Verification items for the finished model (mm, model axes). A direction names the side the tool comes from. Give positions to 0.01 mm unless a question says otherwise; leave off trailing zeros. Write each loop counter-clockwise with the first axis right and the second up, starting at its lowest first coordinate (ties: lowest second). Pieces come first, ordered by that corner, then holes. Notation, with made-up numbers: (57, -37) - (98, -37) arc R22 ccw to (98, -8) - close; hole circle Ø6 at (31, 42.25). An arc over 180 degrees is marked (long way). Put each result on its own line as item: value.
from build123d import *

# Parameters (mm, degrees)
BASPROSKE_W         = 6
BASPROSKE_H         = 8
TOOTHCUT_DEPTH      = 13.806248475
TEETHCUTS_COUNT     = 14
TEETHCUTS_ANGLE     = 334.285714286
BORSKE_R            = 2.5
BORE_DEPTH          = 50.0000508
SKETCH1_R           = 2.5
BOSS_EXTRUDE1_DEPTH = 2.5
SKETCH2_R           = 2.5
CUT_EXTRUDE1_DEPTH  = 1.5
SKETCH3_R           = 1.1
CUT_EXTRUDE2_DEPTH  = 13.073146116


with BuildPart() as part:
    # BasProSke → Base-Revolve (revolve)
    with BuildSketch(Plane(origin=(0, 0, 0), x_dir=(1, 0, 0), z_dir=(0, 1, 0)), mode=Mode.PRIVATE) as base_revolve_sk:
        with Locations((3, 4)):
            Rectangle(BASPROSKE_W, BASPROSKE_H)
    revolve(base_revolve_sk.sketch.rotate(Axis((-10, 0, 0), (1, 0, 0)), 180), axis=Axis((-10, 0, 0), (1, 0, 0)))

    # TooCutSke → ToothCut (cut, through all)
    with BuildSketch(Plane(origin=(0, 0, 0), x_dir=(0, 0, -1), z_dir=(1, 0, 0))):
        with BuildLine():
            ThreePointArc((0.540393256, 5.723545765), (0, 5.749), (-0.540393256, 5.723545765))
            ThreePointArc((-0.540393256, 5.723545765), (-0.832220085, 6.912663993), (-1.603550271, 7.863566092))
            ThreePointArc((-1.603550271, 7.863566092), (0, 8.0254), (1.603550271, 7.863566092))
            ThreePointArc((1.603550271, 7.863566092), (0.832220085, 6.912663993), (0.540393256, 5.723545765))
        make_face()
    toothcut = extrude(amount=TOOTHCUT_DEPTH, mode=Mode.SUBTRACT)

    # TeethCuts: ToothCut ×14 about axis
    teethcuts_axis = Axis((-10, 0, 0), (1, 0, 0))
    for i in range(1, TEETHCUTS_COUNT):
        add(toothcut.rotate(teethcuts_axis, i * TEETHCUTS_ANGLE / (TEETHCUTS_COUNT - 1)), mode=Mode.SUBTRACT)

    # BorSke → Bore (cut, symmetric)
    with BuildSketch(Plane(origin=(0, 0, 0), x_dir=(0, 0, -1), z_dir=(1, 0, 0))):
        with Locations(Location((0, 0, 0), (0, 0, 180))):
            Circle(BORSKE_R)
    extrude(amount=BORE_DEPTH, both=True, mode=Mode.SUBTRACT)

    # Sketch1 → Boss-Extrude1 (add)
    with BuildSketch(Plane(origin=(6, 0, 0), x_dir=(0, 0, -1), z_dir=(1, 0, 0))):
        Circle(SKETCH1_R)
    extrude(amount=-BOSS_EXTRUDE1_DEPTH)

    # Sketch2 → Cut-Extrude1 (cut)
    with BuildSketch(Plane(origin=(6, 0, 0), x_dir=(0, 0, -1), z_dir=(1, 0, 0))):
        Circle(SKETCH2_R)
    extrude(amount=-CUT_EXTRUDE1_DEPTH, mode=Mode.SUBTRACT)

    # Sketch3 → Cut-Extrude2 (cut, through all)
    with BuildSketch(Plane(origin=(4.5, 0, 0), x_dir=(0, 0, -1), z_dir=(1, 0, 0))):
        Circle(SKETCH3_R)
    extrude(amount=-CUT_EXTRUDE2_DEPTH, mode=Mode.SUBTRACT)


solid = part.part
Q1. Scan lines: line 1 along Y through (x, z) = (1.8, 7.25); line 2 along Z through (x, y) = (1.5, 0); line 3 along Z through (x, y) = (1.75, 5.25). Record each from-to range of solid material in increasing order.
Answers follow:
line 1: y = -3.38 to -3.2, -0.63 to 0.63, 3.2 to 3.38
line 2: z = -8 to -2.5, 2.5 to 8
line 3: z = -5 to -3.17, -2.34 to 2.34, 3.17 to 5
Q2. Section check D-D, the plane y = -2. Record the cut outline in (x, z), plus the area to 3 significant figures.
Answers follow:
outline: (0, -6.01) - (6, -6.01) - (6, -1.5) - (4.5, -1.5) - (4.5, 1.5) - (6, 1.5) - (6, 6.01) - (0, 6.01) - (0, 1.5) - (3.5, 1.5) - (3.5, -1.5) - (0, -1.5) - close
area: 57.1 mm2
Q3. Section check B-B, the plane z = 0. Record the cut outline in (x, y), plus the area to 3 significant figures.
Answers follow:
outline: (0, -5.75) - (6, -5.75) - (6, -2.5) - (4.5, -2.5) - (4.5, -1.1) - (3.5, -1.1) - (3.5, -2.5) - (0, -2.5) - close; (0, 2.5) - (3.5, 2.5) - (3.5, 1.1) - (4.5, 1.1) - (4.5, 2.5) - (6, 2.5) - (6, 5.75) - (0, 5.75) - close
area: 41.8 mm2
Q4. Release check for a two-part mould opening along Y. For faces 1 (the face through (2.96, -5.87, 3.75)), 2 (the face through (3, -1.3, 5.6)), 3 (the face through (2.958, 6.882, 0.817)) record: released by +Y, released by -Y, zero draft, split by the parting line, or undercut.
Answers follow:
face 1: released by -Y
face 2: undercut
face 3: released by +Y
Q5. Go/stop test with flat-tipped pins: pin 1 Ø3 at (x, z) = (2.5, 5.5) entering from +Y; pin 2 Ø5.5 at (y, z) = (-1, 1) entering from -X; pin 3 Ø4.5 at (y, z) = (0, 0) entering from -X; pin 4 Ø2 at (x, y) = (5.5, -2.5) entering from +Z. Record where each tip stops, or that it passes through.
Answers follow:
pin 1: stops at y = 6.38
pin 2: stops at x = 0
pin 3: stops at x = 3.5
pin 4: stops at z = 7.3
Q6. Section check C-C, the plane z = -6.5. Record the cut outline in (x, y).
Answers follow:
outline: (0, -3.72) - (6, -3.72) - (6, -2.31) - (0, -2.31) - close; (0, -0.8) - (6, -0.8) - (6, 0.8) - (0, 0.8) - close; (0, 2.31) - (6, 2.31) - (6, 3.72) - (0, 3.72) - close
Q7. Section check A-A, the plane y = 0. Record the cut outline in (x, z), plus the area to 3 significant figures.
Answers follow:
outline: (0, -8) - (6, -8) - (6, -2.5) - (4.5, -2.5) - (4.5, -1.1) - (3.5, -1.1) - (3.5, -2.5) - (0, -2.5) - close; (0, 2.5) - (3.5, 2.5) - (3.5, 1.1) - (4.5, 1.1) - (4.5, 2.5) - (6, 2.5) - (6, 8) - (0, 8) - close
area: 68.8 mm2
Q8. Set-up check for faces 4 (the face through (2.958, 4.961, 4.886)), 5 (the face through (2.96, 6.56, -2.25)), 6 (the face through (2.96, 6.91, -0.83)): record each of +Z, -Z, +X, -X, +Y, -Y from which the full face is reachable in a straight line by a thin tool's end or side.
Answers follow:
face 4: +Z, +X, -X
face 5: +X, -X
face 6: +X, -X, +Y
